Verification items for the finished model (mm, model axes). Face numbers are marked on the shaded views. A direction names the side the tool comes from. Round coordinates to 2 decimals unless told otherwise and drop trailing zeros. Loops run counter-clockwise (first coordinate to the right, second up) from the corner with the lowest first, then second, coordinate; pieces in that order, holes last. Notation, with made-up numbers: (18.5, 84.25) - (65.5, 84.25) arc R17 ccw to (65.5, 102.25) - close; hole circle Ø2 at (30.5, 43.5). An arc over 180 degrees is marked (long way). Use a Markdown table: item, result. Add a question column.
```python
from build123d import *

# Parameters (mm, degrees)
SKETCH_2_W          = 32
SKETCH_2_H          = 40
EXTRUDE_1_DEPTH     = 3
SKETCH_3_W          = 32
SKETCH_3_H          = 3
EXTRUDE_2_DEPTH     = 37
SKETCH_4_R          = 4
SKETCH_4_R_2        = 1.55
SKETCH_4_R_3        = 1.05
CUT_EXTRUDE_1_DEPTH = 57.789083458
SKETCH_6_R          = 2.05
CUT_EXTRUDE_2_DEPTH = 46
FILLET_1_R          = 5
SKETCH_11_R         = 1.55
SKETCH_11_R_2       = 1.05
SKETCH_11_R_3       = 4
EXTRUDE_4_DEPTH     = 1
FILLET_3_R          = 1


with BuildPart() as part:
    # 草图2 → 凸台-拉伸1 (new body)
    with BuildSketch(Plane(origin=(0, 0, 0), x_dir=(1, 0, 0), z_dir=(0, 1, 0))):
        Rectangle(SKETCH_2_W, SKETCH_2_H)
    extrude(amount=EXTRUDE_1_DEPTH)

    # 草图3 → 凸台-拉伸2 (add)
    with BuildSketch(Plane(origin=(0, 3, 0), x_dir=(1, 0, 0), z_dir=(0, 1, 0))):
        with Locations((0, 18.5)):
            Rectangle(SKETCH_3_W, SKETCH_3_H)
    extrude(amount=EXTRUDE_2_DEPTH)

    # 草图4 → 切除-拉伸1 (cut, through all)
    with BuildSketch(Plane.XY.offset(-17)):
        with Locations((0, 20)):
            Circle(SKETCH_4_R)
        with Locations((7, 20)):
            Circle(SKETCH_4_R_2)
        with Locations((0, 13)):
            Circle(SKETCH_4_R_2)
        with Locations((-7, 20)):
            Circle(SKETCH_4_R_2)
        with Locations((0, 27)):
            Circle(SKETCH_4_R_2)
        with Locations((4.949747468, 24.949747468)):
            Circle(SKETCH_4_R_3)
        with Locations((4.949747468, 15.050252532)):
            Circle(SKETCH_4_R_3)
        with Locations((-4.949747468, 15.050252532)):
            Circle(SKETCH_4_R_3)
        with Locations((-4.949747468, 24.949747468)):
            Circle(SKETCH_4_R_3)
    extrude(amount=-CUT_EXTRUDE_1_DEPTH, mode=Mode.SUBTRACT)

    # 草图6 → 切除-拉伸2 (cut, through all)
    with BuildSketch(Plane(origin=(0, 3, 0), x_dir=(1, 0, 0), z_dir=(0, 1, 0))):
        with Locations(Location((0, -5, 0), (0, 0, 270))):
            Circle(SKETCH_6_R)
        with Locations(Location((-8, -5, 0), (0, 0, 270))):
            Circle(SKETCH_6_R)
        with Locations(Location((8, -5, 0), (0, 0, 270))):
            Circle(SKETCH_6_R)
        with Locations(Location((0, 3, 0), (0, 0, 270))):
            Circle(SKETCH_6_R)
        with Locations(Location((0, -13, 0), (0, 0, 270))):
            Circle(SKETCH_6_R)
    extrude(amount=-CUT_EXTRUDE_2_DEPTH, mode=Mode.SUBTRACT)

    # 圆角1
    fillet_1_edges = [part.edges().sort_by_distance(p)[0] for p in [
        (-16, 40, -18.5),
        (16, 40, -18.5),
        (16, 1.5, 20),
        (-16, 1.5, 20),
    ]]
    fillet(fillet_1_edges, radius=FILLET_1_R)

    # 草图11 → 凸台-拉伸4 (add)
    with BuildSketch(Plane(origin=(0, 0, -20), x_dir=(-1, 0, 0), z_dir=(0, 0, -1))):
        with BuildLine():
            Line((11, 40), (-11, 40))
            ThreePointArc((-11, 40), (-14.535533906, 38.535533906), (-16, 35))
            Line((-16, 35), (-16, 0))
            Line((-16, 0), (16, 0))
            Line((16, 0), (16, 35))
            ThreePointArc((16, 35), (14.535533906, 38.535533906), (11, 40))
        make_face()
        with Locations(Location((-7, 20, 0), (0, 0, 180))):
            Circle(SKETCH_11_R, mode=Mode.SUBTRACT)
        with Locations(Location((-4.949747468, 15.050252532, 0), (0, 0, 180))):
            Circle(SKETCH_11_R_2, mode=Mode.SUBTRACT)
        with Locations(Location((0, 13, 0), (0, 0, 180))):
            Circle(SKETCH_11_R, mode=Mode.SUBTRACT)
        with Locations(Location((0, 20, 0), (0, 0, 180))):
            Circle(SKETCH_11_R_3, mode=Mode.SUBTRACT)
        with Locations(Location((4.949747468, 15.050252532, 0), (0, 0, 180))):
            Circle(SKETCH_11_R_2, mode=Mode.SUBTRACT)
        with Locations(Location((7, 20, 0), (0, 0, 180))):
            Circle(SKETCH_11_R, mode=Mode.SUBTRACT)
        with Locations(Location((4.949747468, 24.949747468, 0), (0, 0, 180))):
            Circle(SKETCH_11_R_2, mode=Mode.SUBTRACT)
        with Locations(Location((-4.949747468, 24.949747468, 0), (0, 0, 180))):
            Circle(SKETCH_11_R_2, mode=Mode.SUBTRACT)
        with Locations(Location((0, 27, 0), (0, 0, 180))):
            Circle(SKETCH_11_R, mode=Mode.SUBTRACT)
    extrude(amount=EXTRUDE_4_DEPTH)

    # 圆角3
    fillet_3_edges = [part.edges().sort_by_distance(p)[0] for p in [
        (0, 0, -21),
    ]]
    fillet(fillet_3_edges, radius=FILLET_3_R)


solid = part.part
```
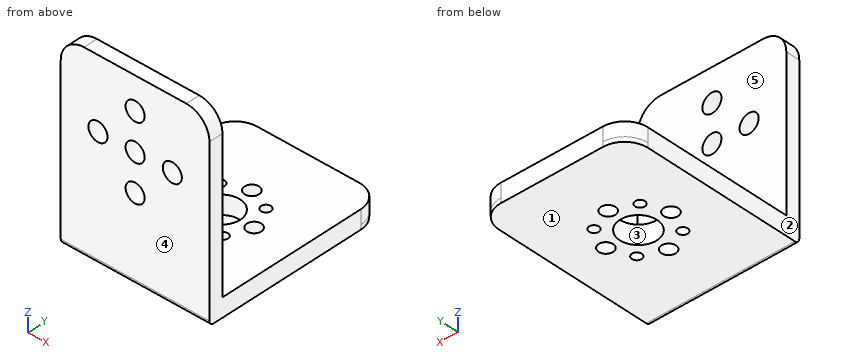
Q1. Section check D-D on x = -7. Record the cut outline in (y, z).
Q2. Set-up check for the marked faces 4 and 5: record each of +Z, -Z, +X, -X, +Y, -Y from which the full face is reachable in a straight line by a thin tool's end or side.
Q3. Release check for a two-part mould opening along X. For the marked faces 1, 2 and 3 record: +X half, -X half, draft (parallel to the pull), parting line (faces both ways), or undercut.
Q4. Thickness scan on line 1 along X through (y, z) = (1, 5); line 2 along X through (y, z) = (20, -18.2); line 3 along Y through (x, z) = (6, -7). Record the ranges inside material, lowest first.
Q5. Go/stop test with flat-tipped pins: pin 1 Ø3.5 at (x, y) = (-4.95, 24.95) entering from +Z; pin 2 Ø1.9 at (x, y) = (4.95, 24.95) entering from -Z; pin 3 Ø16 at (x, z) = (-4, 3) entering from +Y. Record where each tip stops, or that it passes through.
Q6. Section check A-A on x = 0. State how many separate pieces and enclosed holes the cut face has, plus the area to 3 significant figures.
Q7. Section check C-C on y = 13. Record the cut outline in (x, z), plus the area to 3 significant figures.
Q8. Section check B-B on z = -3. Record the cut outline in (x, y).
Determined:
| question | item | result |
|---|---|---|
| 1 | outline | (0, -20) arc R1 ccw to (1, -21) - (18.45, -21) - (18.45, -17) - (3, -17) - (3, 3.21) - (0, 3.21) - close; (0, 6.79) - (3, 6.79) - (3, 20) - (0, 20) - close; (21.55, -21) - (40, -21) - (40, -17) - (21.55, -17) - close |
| 2 | face 4 | +Z, -Z, +X, -X, -Y |
| 2 | face 5 | +Z, +X, -X, +Y |
| 3 | face 1 | draft |
| 3 | face 2 | -X half |
| 3 | face 3 | undercut |
| 4 | line 1 | x = -16 to -10.05, -5.95 to -2.05, 2.05 to 5.95, 10.05 to 16 |
| 4 | line 2 | x = -16 to -8.55, -5.45 to -4, 4 to 5.45, 8.55 to 16 |
| 4 | line 3 | y = 0 to 3 |
| 5 | pin 1 | stops at z = -17 |
| 5 | pin 2 | passes through |
| 5 | pin 3 | stops at y = 3 |
| 6 | separate pieces | 7 |
| 6 | enclosed holes | 0 |
| 6 | area | 177 mm² |
| 7 | outline | (-16, -21) - (-1.55, -21) - (-1.55, -17) - (-16, -17) - close; (1.55, -21) - (16, -21) - (16, -17) - (1.55, -17) - close |
| 7 | area | 116 mm² |
| 8 | outline | (-16, 0) - (-2.05, 0) - (-2.05, 3) - (-16, 3) - close; (2.05, 0) - (16, 0) - (16, 3) - (2.05, 3) - close |
